Model file for the job. Use its own axes, mm. A direction names the side the tool comes from. Give positions to 0.01 mm unless a question says otherwise; leave off trailing zeros. Order: outer loops, then holes, each group sorted by start corner. A loop starts at its lowest first (then second) coordinate and runs counter-clockwise, first axis right, second up. Notation, with made-up numbers: (14.5, 0) -> (18.5, 0) arc R30 cw to (18.5, 23) -> close; hole circle Ø9 at (51, -25). An arc over 180 degrees is marked (long way). Use CSV: the item, a comma, the result in double quotes. Start each with the question number.
1. Pull direction X, two halves, no side cores. Call faces 1 (the cylindrical face through (7.05, 66.07, 9.76)), 2 (the flat face through (21, 66, 15.875)), 3 (the cylindrical face through (1.91, 74.84, 3.22)): released by +X, released by -X, zero draft, split by the parting line, or undercut.
2. 3-axis set-ups, long thin cutter, end or side, ignore diameter. For faces 4 (the flat face through (23, 68.488, 11)), 5 (the cylindrical face through (36.338, 66.073, 9.593)), 6 (the flat face through (17, 76.651, 3)), 7 (the cylindrical face through (59.717, 86.852, 12.611)): which of +Z, -Z, +X, -X, +Y, -Y reach the whole face in a straight line?
3. Cut at B-B on y = 94.5. List the corners of the cut face in (x, z).
4. Cut at C-C on x = 53.5. List the corners of the cut face in (y, z), then the cut area to 3 significant figures.
5. Drop flat-ended pins along their axis: pin 1 (3 mm diameter, centred on y = 72.5, z = 7.5, fed in from +X); pin 2 (7 mm diameter, centred on x = 9.04, z = 10.8, fed in from +Y); pin 3 (10 mm diameter, centred on x = 33, y = 74.5, fed in from +Z). Give the stop position or say it passes through.
6. Wall check: line 1 (Z direction, x = 22, y = 72); line 2 (Y direction, x = 24.5, z = 7); line 3 (Z direction, x = 16, y = 68) (3 decimals). Give the ranges that are in metal, low to high. Write a range as from..to.
7. Cut at D-D on z = 17.5. List the corners of the cut face in (x, y).
Autodesk Inventor part; units mm, degrees
ref_plane "Work Plane1" through (0, 38.3255, 0) normal (0, 1, 0) x (1, 0, 0)
ref_plane "YZ Plane" through (0, 0, 0) normal (1, 0, 0) x (0, 1, 0)
ref_plane "XZ Plane" through (0, 0, 0) normal (0, 1, 0) x (-1, 0, 0)
sketch "Sketch1" plane through (0, 0, 0) normal (0, 0, 1) x (1, 0, 0)
  line L0 (0, 0) -> (63.5, 0)
  line L1 (63.5, 0) -> (63.5, 12.9255)
  line L2 (63.5, 12.9255) -> (0, 12.9255)
  line L3 (0, 12.9255) -> (0, 0)
  line L4 (63.5, 12.9255) -> (50.8, 12.9255)
  line L5 (50.8, 12.9255) -> (50.8, -19.0013)
  line L6 (50.8, -19.0013) -> (63.5, -19.0013)
  line L7 (63.5, -19.0013) -> (63.5, 12.9255)
  point P0 (57.15, -14.2271)
  point P1 (34.4424, 12.9255)
  point P2 (9.0424, 12.9255)
  dimension "d0" = 63.5
  dimension "d2" = 22.7076
  dimension "d3" = 25.4
  dimension "d4" = 27.1526
  dimension "d5" = 0
  dimension "d6" = 6.35
  dimension "d7" = 6.35
extrude "Extrusion1" add sketch "Sketch1" along normal blind 6.35
sketch "Sketch2" plane through (0, 0, 6.35) normal (0, 0, 1) x (1, 0, 0)
  line L0 (63.5, -19.0013) -> (63.5, 12.9255)
  line L1 (50.8, 0) -> (50.8, -19.0013)
  line L2 (63.5, 12.9255) -> (0, 12.9255)
  point P0 (0, 0)
  point P1 (57.15, -14.2271)
  dimension "d10" = 6.35
  dimension "d11" = 6.35
  dimension "d12" = 27.1526
hole "Hole1" at (57.15, -14.2271, 6.35) direction (0, 0, -1) diameter 5.5 depth 25.4 tip angle 118
sketch "Sketch3" plane through (0, 0, 6.35) normal (0, 0, 1) x (1, 0, 0)
  circle A0 centre (57.15, -14.2271) radius 2.75
  circle A1 centre (57.15, -14.2271) radius 4.7742
  line L0 (50.8, -19.0013) -> (63.5, -19.0013)
  point P0 (0, 0)
extrude "Extrusion2" add sketch "Sketch3" along normal blind 12.7
fillet "Fillet1" radius 6.35 2 edges at (63.5, -19.0013, 3.175) (50.8, -19.0013, 3.175)
fillet "Fillet2" radius 25.4 2 edges at (50.8, 0, 3.175) (63.5, 12.9255, 3.175)
sketch "Sketch4" plane through (0, 0, 6.35) normal (0, 0, 1) x (1, 0, 0)
  line L0 (0, 12.9255) -> (0, 0)
  line L1 (0, 12.9255) -> (40.7924, 12.9255)
  line L2 (40.7924, 12.9255) -> (40.7924, 8.163)
  line L3 (40.7924, 8.163) -> (0, 8.163)
  line L4 (0, 8.163) -> (0, 12.9255)
  circle A0 centre (57.15, -14.2271) radius 2.75
  dimension "d24" = 16.3576
  dimension "d25" = 4.7625
extrude "Extrusion3" add sketch "Sketch4" along normal blind 9.525 contours L1 L2 L3 L0
fillet "Fillet3" radius 6.35 2 edges at (40.7924, 10.5443, 15.875) (0, 10.5443, 15.875)
fillet "Fillet4" radius 6.35 1 edges at (40.7924, 10.4727, 6.35)
sketch "Sketch5" plane through (6.35, 8.163, 15.875) normal (0, -1, 0) x (1, 0, 0)
  line L0 (48.05, 3.175) -> (53.55, 3.175)
  point P0 (-6.35, -15.875)
  point P1 (2.6924, -5.0739)
  point P2 (28.0924, -5.0739)
  point P3 (50.8, 3.175)
  dimension "d30" = 25.4
  dimension "d31" = 22.7076
hole "Hole2" at (9.0424, 8.163, 10.8011) at (34.4424, 8.163, 10.8011) at (57.15, 8.163, 19.05) direction (0, 1, 0) diameter 4.4958 depth 25.4 tip angle 118
fillet "Fillet5" radius 6.35 1 edges at (0, 0, 3.175)
ref_plane "Work Plane1" through (0, 38.3255, 0) normal (0, 1, 0) x (1, 0, 0)
mirror "Mirror1" about plane through (0, 38.3255, 0) normal (0, 1, 0) of "Extrusion3", "Fillet4", "Fillet5", "Hole2", "Fillet3", "Fillet2", "Fillet1", "Extrusion2", "Hole1", "Extrusion1"
sketch "Sketch6" plane through (0, 12.9255, 0) normal (0, 1, 0) x (1, 0, 0)
  line L0 (75.6078, -32.1869) -> (-9.353, -32.1869)
  line L1 (-9.353, -32.1869) -> (-9.353, 6.0612)
  line L2 (-9.353, 6.0612) -> (75.6078, 6.0612)
  line L3 (75.6078, 6.0612) -> (75.6078, -32.1869)
  point P0 (0, 0)
extrude "Extrusion4" cut sketch "Sketch6" against normal blind 101.6
properties part number "supporty2"
Verdict:
1,face 1,"undercut"
1,face 2,"zero draft"
1,face 3,"released by -X"
2,face 4,"+Z, +X, -X, +Y"
2,face 5,"+Y, -Y"
2,face 6,"+Z, -Z, -X, +Y"
2,face 7,"+Z"
3,outline,"(53.5, 0) -> (60.8, 0) -> (60.8, 6.35) -> (60.26, 6.35) -> (60.26, 19.05) -> (54.04, 19.05) -> (54.04, 6.35) -> (53.5, 6.35) -> close"
4,outline,"(68.93, 0) -> (94.5, 0) -> (94.5, 6.35) -> (93.96, 6.35) -> (93.96, 19.05) -> (87.8, 19.05) -> (87.8, 6.35) -> (68.93, 6.35) -> close"
4,area,"241 mm^2"
5,pin 1,"x = 58.1"
5,pin 2,"y = 68.49"
5,pin 3,"z = 6.35"
6,line 1,"0..6.35"
6,line 2,"63.73..68.49"
6,line 3,"0..15.875"
7,outline,"circle Ø9.55 at (57.15, 90.88); hole circle Ø5.5 at (57.15, 90.88)"
